from build123d import *

# Parameters (mm, degrees)
F0_R     = 1.9812
F1_DEPTH = 7.5057
F3_DEPTH = 1.7526
F4_W     = 7.3152
F4_H     = 1.5748
F5_DEPTH = 2.159
F6_R     = 0.79375


with BuildPart() as f1:
    # F0 (on Top) → F1 (new body, symmetric)
    with BuildSketch(Plane.XY):
        Circle(F0_R)
    extrude(amount=F1_DEPTH, both=True)

    # F2 (on Top) → F3 (join, symmetric)
    with BuildSketch(Plane.XY):
        Polygon((1.871663, 0.649638), (-1.871663, 0.649638), (-3.6576, -4.4958), (0, -4.4958), (3.6576, -4.4958), align=None)
    extrude(amount=F3_DEPTH, both=True)

    # F4 (on face) → F5 (cut)
    with BuildSketch(Plane.XZ.offset(4.4958)):
        Rectangle(F4_W, F4_H)
    extrude(amount=-F5_DEPTH, mode=Mode.SUBTRACT)

    # F6
    f6_edges = [f1.edges().sort_by_distance(p)[0] for p in [
        (-1.9812, 0, 7.5057),
        (-1.9812, 0, -7.5057),
    ]]
    fillet(f6_edges, radius=F6_R)


solid = f1.part
Read the model definition and answer for the solid it produces. Units are mm, in the model's axes. A direction names the side the tool comes from. Coordinates: 2 decimals unless noted, no trailing zeros. Write each loop counter-clockwise with the first axis right and the second up, starting at its lowest first coordinate (ties: lowest second). Pieces come first, ordered by that corner, then holes. Notation, with made-up numbers: M 15.5,-38 L 40.5,-38 A21 ccw 40.5,-23 Z; hole C -8.75,-29.75 d2. An arc over 180 degrees is marked long. Use a Markdown table: item, result.
Q1. Each of these flat-tipped pins is pushed along its axis until it touches: pin 1 Ø1.5 at (x, z) = (-2.5, 5) entering from +Y; pin 2 Ø2 at (y, z) = (0, 1) entering from +X; pin 3 Ø1 at (y, z) = (-2, -1) entering from -X. Where does it stop, or does it pass through?
Answer block:
| item | result |
|---|---|
| pin 1 | stops at y = 0.93 |
| pin 2 | stops at x = 2.44 |
| pin 3 | stops at x = -2.96 |
Q2. The part is cut by section A-A, the plane x = 3.25. Write down the section's boundary in (y, z), then the cut area to 3 significant figures.
Answer block:
| item | result |
|---|---|
| outline | M -4.5,-1.75 L -3.32,-1.75 L -3.32,-0.79 L -4.5,-0.79 Z; M -4.5,0.79 L -3.32,0.79 L -3.32,1.75 L -4.5,1.75 Z |
| area | 2.27 mm2 |
Q3. Straight lines are drawn through the part: L1, parallel to Z at x = -0.25, y = -4; L2, parallel to Y at x = 0.5, z = -5; L3, parallel to X at y = -1, z = 4.75. For each, find the intervals that lie inside material, in ascending order. Write a range as [from, to].
Answer block:
| item | result |
|---|---|
| L1 | z = [-1.75, -0.79], [0.79, 1.75] |
| L2 | y = [-1.92, 1.92] |
| L3 | x = [-1.71, 1.71] |
Q4. The part is cut by section C-C, the plane x = 0. Write down the section's boundary in (y, z).
Answer block:
| item | result |
|---|---|
| outline | M -4.5,-1.75 L -1.98,-1.75 L -1.98,-6.71 A0.79 ccw -1.19,-7.51 L 1.19,-7.51 A0.79 ccw 1.98,-6.71 L 1.98,6.71 A0.79 ccw 1.19,7.51 L -1.19,7.51 A0.79 ccw -1.98,6.71 L -1.98,1.75 L -4.5,1.75 L -4.5,0.79 L -2.34,0.79 L -2.34,-0.79 L -4.5,-0.79 Z |
Q5. Determine the mould class of faces 4 (the face through (2.58, -1.39, 0.02)), 5 (the face through (0, -3, -1.753)), 6 (the face through (0, -3, -0.787)) for opening direction Z: released by +Z, released by -Z, zero draft, split by the parting line, or undercut.
Answer block:
| item | result |
|---|---|
| face 4 | zero draft |
| face 5 | released by -Z |
| face 6 | undercut |
Q6. Which of the six approach directions +Z, -Z, +X, -X, +Y, -Y give full straight-line access (tool end or side, diameter ignored) to faces 1 (the face through (0, -4.496, 1)), 2 (the face through (-0.258, 1.964, 0.094)), 3 (the face through (0, -2.337, 0))?
Answer block:
| item | result |
|---|---|
| face 1 | +Z, -Z, +X, -X, -Y |
| face 2 | none |
| face 3 | +X, -X, -Y |
Q7. The part is cut by section B-B, the plane y = -3. Write down the section's boundary in (x, z), then the cut area to 3 significant figures.
Answer block:
| item | result |
|---|---|
| outline | M -3.14,-1.75 L 3.14,-1.75 L 3.14,-0.79 L -3.14,-0.79 Z; M -3.14,0.79 L 3.14,0.79 L 3.14,1.75 L -3.14,1.75 Z |
| area | 12.1 mm2 |
Q8. The part is cut by section D-D, the plane z = -0.5. Write down the section's boundary in (x, y).
Answer block:
| item | result |
|---|---|
| outline | M -2.91,-2.34 L 2.91,-2.34 L 1.87,0.65 A1.98 ccw -1.87,0.65 Z |
